Autodesk Inventor part; units mm, degrees
ref_plane "YZ Plane" through (0, 0, 0) normal (1, 0, 0) x (0, 1, 0)
ref_plane "XZ Plane" through (0, 0, 0) normal (0, 1, 0) x (-1, 0, 0)
ref_plane "XY Plane" through (0, 0, 0) normal (0, 0, 1) x (1, 0, 0)
sketch "Sketch1" plane through (0, 0, 0) normal (1, 0, 0) x (0, 1, 0)
  line L0 (0, 0) -> (25.4, 0)
  line L1 (25.4, 0) -> (25.4, -64.6049)
  line L2 (25.4, -64.6049) -> (0, -64.6049)
  line L3 (0, -64.6049) -> (0, 0)
  line L4 (0, -3.175) -> (22.225, -3.175)
  line L5 (22.225, -3.175) -> (22.225, -61.4299)
  line L6 (22.225, -61.4299) -> (0, -61.4299)
  line L7 (0, -61.4299) -> (0, -3.175)
  dimension "d0" = 25.4
  dimension "d2" = 58.2549
  dimension "d3" = 22.225
  dimension "d4" = 3.175
  dimension "d32" = 3.175
extrude "Extrusion1" add sketch "Sketch1" along normal blind 495.3 contours L0 L1 L2 L3 L6 L5 L4
sketch "Sketch3" plane through (0, 25.4, 0) normal (0, 1, 0) x (1, 0, 0)
  line L0 (0, 64.6049) -> (0, 0)
  line L1 (0, 0) -> (495.3, 0)
  line L2 (495.3, 64.6049) -> (495.3, 0)
  line L3 (0, 64.6049) -> (495.3, 64.6049)
  line L4 (495.3, 3.175) -> (457.2, 3.175)
  line L5 (457.2, 3.175) -> (457.2, 61.4299)
  line L6 (457.2, 61.4299) -> (495.3, 61.4299)
  line L7 (495.3, 61.4299) -> (495.3, 3.175)
  line L8 (0, 64.6049) -> (0, 0)
  line L9 (0, 3.175) -> (38.1, 3.175)
  line L10 (38.1, 3.175) -> (38.1, 61.4299)
  line L11 (38.1, 61.4299) -> (0, 61.4299)
  line L12 (0, 61.4299) -> (0, 3.175)
  point P0 (495.3, 61.4299)
  dimension "d14" = 64.6049
  dimension "d16" = 38.1
  dimension "d27" = 38.1
  dimension "d28" = 58.2549
  dimension "d29" = 3.175
  dimension "d30" = 58.2549
  dimension "d31" = 3.175
extrude "Extrusion2" cut sketch "Sketch3" against normal blind 3.175 contours L11 L10 L9 L0 | L2 L4 L5 L6
sketch "Sketch4" plane through (0, 0, 0) normal (0, 0, 1) x (1, 0, 0)
  line L0 (0, 25.4) -> (0, 0)
  line L1 (0, 0) -> (495.3, 0)
  line L2 (495.3, 25.4) -> (495.3, 0)
  line L3 (0, 25.4) -> (495.3, 25.4)
  circle A0 centre (12.7, 12.7) radius 3.175
  circle A1 centre (482.6, 12.7) radius 3.175
  dimension "d19" = 6.35
  dimension "d20" = 12.7
  dimension "d21" = 25.4
  dimension "d22" = 12.7
  dimension "d23" = 6.35
  dimension "d24" = 12.7
extrude "Extrusion3" cut sketch "Sketch4" against normal blind 127 contours A0 | A1
equation "\"d32\" = d4"
equation "\"d30\" = d28"
equation "\"d31\" = d29"
equation "\"d22\" = 0.5 * d21"
equation "\"d23\" = d19"
equation "\"d24\" = d20"
properties part number "ArmProto2.2Assembly"
Geometry check sheet. Reference: the model listing, model coordinates, mm. A direction names the side the tool comes from. Round coordinates to 2 decimals unless told otherwise and drop trailing zeros. Loops run counter-clockwise (first coordinate to the right, second up) from the corner with the lowest first, then second, coordinate; pieces in that order, holes last.
Item 1: Access from +Z, -Z, +X, -X, +Y, -Y to the whole of each face (thin tool, end or side, straight path). Record for faces 1 (the flat face through (244, 13, 0)), 2 (the flat face through (245, 22.225, -32)).
Item 2: Mould release check, pull along Z, two halves, no side actions. Record for faces 3 (the flat face through (244, 13, -3.175)), 4 (the flat face through (244, 13, -64.605)), 5 (the flat face through (244, 25.4, -32)): pulls with the +Z half, pulls with the -Z half, needs draft (parallel to the pull), parting line crosses it, or undercut.
Item 3: Cross-section at B-B on z = -38. Record the boundary of the cut face in (x, y) (3 decimals), then the cut area to 3 significant figures.
Item 4: Gauge pin test, flat ends, axial feed: pin 1 (1.6 mm diameter, centred on y = 24, z = -40, fed in from +X); pin 2 (8.5 mm diameter, centred on x = 482.6, y = 12.7, fed in from +Z); pin 3 (1 mm diameter, centred on x = 273, z = -45.5, fed in from -Y) (3 decimals); pin 4 (5 mm diameter, centred on x = 482.6, y = 12.7, fed in from -Z). Record the tip position at first contact, or that the pin passes through.
Item 5: Cross-section at A-A on x = 410.5. Record the boundary of the cut face in (y, z) (3 decimals), then the cut area to 3 significant figures.
Item 6: Thickness scan on line 1 (Z direction, x = 364.5, y = 1.5) (3 decimals); line 2 (Y direction, x = 12, z = -63); line 3 (Y direction, x = 12.7, z = -1.85) (3 decimals). Record the ranges inside material, lowest first.
Answer sheet:
1. face 1: +Z, +X, -X, +Y, -Y
1. face 2: +X, -X, -Y
2. face 3: undercut
2. face 4: pulls with the -Z half
2. face 5: needs draft
3. outline: (38.1, 22.225) - (457.2, 22.225) - (457.2, 25.4) - (38.1, 25.4) - close
3. area: 1,330 mm2
4. pin 1: stops at x = 457.2
4. pin 2: stops at z = 0
4. pin 3: stops at y = 22.225
4. pin 4: passes through
5. outline: (0, -64.605) - (25.4, -64.605) - (25.4, 0) - (0, 0) - (0, -3.175) - (22.225, -3.175) - (22.225, -61.43) - (0, -61.43) - close
5. area: 346 mm2
6. line 1: z = -64.605 to -61.43, -3.175 to 0
6. line 2: y = 0 to 9.6, 15.8 to 25.4
6. line 3: y = 0 to 9.525, 15.875 to 25.4
